```python
from build123d import *

# Parameters (mm, degrees)
MODEL_R         = 2.032
MODEL_R_2       = 3.048
MODEL_R_3       = 1
MODEL_W         = 13.99947
MODEL_H         = 13.99944
MODEL_W_2       = 13.9993
MODEL_H_2       = 13.9993
MODEL_W_3       = 13.9994
MODEL_W_4       = 2.54
MODEL_H_3       = 3.556
EXTRUDE_1_DEPTH = 1.6


with BuildPart() as part:
    # Model → 凸台-拉伸1 (new body)
    with BuildSketch(Plane.XY):
        Polygon((-4.883883532, 35.973891408), (-4.813241799, 36.606032798), (-4.68610198, 37.230158431), (-4.516543388, 37.837883816), (-4.295846464, 38.426181173), (-4.040425316, 38.98432755), (-3.734657976, 39.530581217), (-3.38546168, 40.058138925), (-2.991401911, 40.556139441), (-2.564669958, 41.019308228), (-2.102117382, 41.445002794), (-1.607054067, 41.836688867), (-1.079854091, 42.186395311), (-0.531138892, 42.493537781), (0.027842562, 42.749214223), (0.615268756, 42.969285901), (1.221866946, 43.138689477), (1.847538347, 43.266199966), (2.481438717, 43.33682275), (2.994321582, 43.3575), (54.345328535, 43.3575), (54.861412529, 43.336821814), (55.491753218, 43.266152175), (56.117576842, 43.139310654), (56.726490724, 42.969125656), (57.312630049, 42.749556004), (57.878545004, 42.490950339), (58.425461808, 42.18272689), (58.9399975, 41.841630195), (59.445802193, 41.444115049), (59.912079101, 41.011414411), (60.332093164, 40.555391632), (60.716064737, 40.069904287), (61.069053534, 39.543781609), (61.382985177, 38.982666106), (61.644423874, 38.410551538), (61.855071366, 37.838089056), (62.028284371, 37.232642984), (62.152332548, 36.60558626), (62.225027392, 35.986226197), (62.246303139, 35.458587663), (58.746175407, 31.358234918), (58.745975132, 24.929084585), (62.245861062, 21.267199282), (62.245579127, 18.534705638), (58.745666056, 15.007268129), (58.745412398, 6.86443549), (62.245297192, 3.166071528), (62.226202972, 2.636734827), (62.152356641, 2.011350393), (62.029241049, 1.384922025), (61.855333273, 0.776565869), (61.644240363, 0.202684675), (61.379380282, -0.376374826), (61.064717919, -0.934798534), (60.721224007, -1.446690794), (60.332973054, -1.941418241), (59.905767444, -2.401934126), (59.445938304, -2.8287768), (58.947571314, -3.220379587), (58.434482529, -3.563431063), (57.880206411, -3.875955859), (57.302144081, -4.140491025), (56.726168878, -4.352867841), (56.11599848, -4.526806688), (55.492240411, -4.649391053), (54.87843401, -4.722059086), (54.34686609, -4.743685), (2.992774524, -4.743685), (2.464503115, -4.722060038), (1.847223482, -4.64943937), (1.223529929, -4.526191258), (0.615600502, -4.353028424), (0.038326794, -4.140153507), (-0.532800957, -3.878547051), (-1.088890304, -3.567123565), (-1.614610519, -3.215411153), (-2.102251702, -2.829663369), (-2.558331876, -2.409802006), (-2.992281832, -1.942165148), (-3.390574278, -1.434889052), (-3.730362364, -0.921623746), (-4.03681533, -0.378036856), (-4.295659415, 0.187060206), (-4.516803943, 0.776764684), (-4.687062167, 1.387481119), (-4.813264805, 2.011073476), (-4.883883595, 2.639206616), (-4.9049154, 3.15597541), (-4.9049154, 4.538497879), (-1.354024868, 8.929084585), (-1.353649461, 15.358051679), (-4.853710523, 19.020120221), (-4.853428588, 21.752613865), (-1.353515518, 25.280051374), (-1.35326186, 33.422884013), (-4.9049154, 35.460217069), align=None)
        with Locations((38.1958, 28.832)):
            Circle(MODEL_R, mode=Mode.SUBTRACT)
        with Locations((19.1458, 28.832)):
            Circle(MODEL_R, mode=Mode.SUBTRACT)
        with Locations((28.6708, 28.832)):
            Circle(MODEL_R_2, mode=Mode.SUBTRACT)
        with Locations((-2.255498735, 20.010211418)):
            Circle(MODEL_R_3, mode=Mode.SUBTRACT)
        with Locations((-1.255498735, 39.010211418)):
            Circle(MODEL_R_3, mode=Mode.SUBTRACT)
        with Locations((57.744501265, 40.010211418)):
            Circle(MODEL_R_3, mode=Mode.SUBTRACT)
        with Locations((59.944501265, 20.010211418)):
            Circle(MODEL_R_3, mode=Mode.SUBTRACT)
        with Locations((8.744501265, -2.189788582)):
            Circle(MODEL_R_3, mode=Mode.SUBTRACT)
        with Locations((48.744501265, -2.189788582)):
            Circle(MODEL_R_3, mode=Mode.SUBTRACT)
        with Locations((9.620765, 9.78198)):
            Rectangle(MODEL_W, MODEL_H, mode=Mode.SUBTRACT)
        with Locations((47.72075, 28.83195)):
            Rectangle(MODEL_W_2, MODEL_H_2, mode=Mode.SUBTRACT)
        with Locations((28.6707, 9.78198)):
            Rectangle(MODEL_W_3, MODEL_H, mode=Mode.SUBTRACT)
        with Locations((9.620765, 28.83195)):
            Rectangle(MODEL_W, MODEL_H_2, mode=Mode.SUBTRACT)
        with Locations((47.72075, 9.78198)):
            Rectangle(MODEL_W_2, MODEL_H, mode=Mode.SUBTRACT)
        with Locations((19.151523106, 9.728566018)):
            Rectangle(MODEL_W_4, MODEL_H_3, mode=Mode.SUBTRACT)
    extrude(amount=EXTRUDE_1_DEPTH)


solid = part.part
```
For this review, take the finished solid that the model builds, in its own axes (mm). A direction names the side the tool comes from. Round coordinates to 2 decimals unless told otherwise and drop trailing zeros. Write each loop counter-clockwise with the first axis right and the second up, starting at its lowest first coordinate (ties: lowest second). Pieces come first, ordered by that corner, then holes. Notation, with made-up numbers: (-6, 89.5) - (18, 89.5) arc R33 ccw to (18, 118.5) - close; hole circle Ø10 at (56, -25.5). An arc over 180 degrees is marked (long way). Answer as a JSON object with one key per item and string values.
1. We need section D-D on y = 13.5. Give the boundary of the cut face in (x, z), then the cut area to 3 significant figures.
Response values:
{"outline": "(-1.35, 0) - (2.62, 0) - (2.62, 1.6) - (-1.35, 1.6) - close; (16.62, 0) - (21.67, 0) - (21.67, 1.6) - (16.62, 1.6) - close; (35.67, 0) - (40.72, 0) - (40.72, 1.6) - (35.67, 1.6) - close; (54.72, 0) - (58.75, 0) - (58.75, 1.6) - (54.72, 1.6) - close", "area": "29.0 mm2"}
2. Tool access review of faces 1 (the face through (60.52, 16.796, 0.789)), 2 (the face through (-3.104, 34.427, 0.789)), 3 (the face through (16.62, 10, 1)): name each direction out of +Z, -Z, +X, -X, +Y, -Y from which nothing blocks a thin tool from reaching the whole face with its end or side.
Response values:
{"face 1": "+Z, -Z, +X", "face 2": "+Z, -Z, -X", "face 3": "+Z, -Z"}
3. Draft analysis for pull direction Y (two halves, no side actions). For faces 4 (the face through (29, 20, 0)), 5 (the face through (-3.079, 17.163, 0.789)), state which applies: +Y half, -Y half, draft (parallel to the pull), parting line (faces both ways), or undercut.
Response values:
{"face 4": "draft", "face 5": "undercut"}
4. We need section C-C on y = 34.5. Give the boundary of the cut face in (x, z), then the cut area to 3 significant figures.
Response values:
{"outline": "(-3.23, 0) - (2.62, 0) - (2.62, 1.6) - (-3.23, 1.6) - close; (16.62, 0) - (40.72, 0) - (40.72, 1.6) - (16.62, 1.6) - close; (54.72, 0) - (61.43, 0) - (61.43, 1.6) - (54.72, 1.6) - close", "area": "58.7 mm2"}
5. To check wall thickness, follow line 1 along Y through (x, z) = (42, 0.6); line 2 along Y through (x, z) = (28.5, 0.5); line 3 along X through (y, z) = (14, 0.9). State the ranges of each line that lie inside material, in increasing order.
Response values:
{"line 1": "y = -4.74 to 2.78, 16.78 to 21.83, 35.83 to 43.36", "line 2": "y = -4.74 to 2.78, 16.78 to 25.79, 31.88 to 43.36", "line 3": "x = -1.35 to 2.62, 16.62 to 21.67, 35.67 to 40.72, 54.72 to 58.75"}
6. We need section B-B on x = 35. Give the boundary of the cut face in (y, z).
Response values:
{"outline": "(-4.74, 0) - (2.78, 0) - (2.78, 1.6) - (-4.74, 1.6) - close; (16.78, 0) - (43.36, 0) - (43.36, 1.6) - (16.78, 1.6) - close"}
7. We need section A-A on x = 46.5. Give the boundary of the cut face in (y, z), then the cut area to 3 significant figures.
Response values:
{"outline": "(-4.74, 0) - (2.78, 0) - (2.78, 1.6) - (-4.74, 1.6) - close; (16.78, 0) - (21.83, 0) - (21.83, 1.6) - (16.78, 1.6) - close; (35.83, 0) - (43.36, 0) - (43.36, 1.6) - (35.83, 1.6) - close", "area": "32.2 mm2"}
